Could you check a few things on this drawing? It's one solid part, dimensions in mm from its lowest x, y, z. A direction names the side the tool comes from. Give positions to 0.01 mm unless a question says otherwise; leave off trailing zeros. Order: outer loops, then holes, each group sorted by start corner. A loop starts at its lowest first (then second) coordinate and runs counter-clockwise, first axis right, second up.
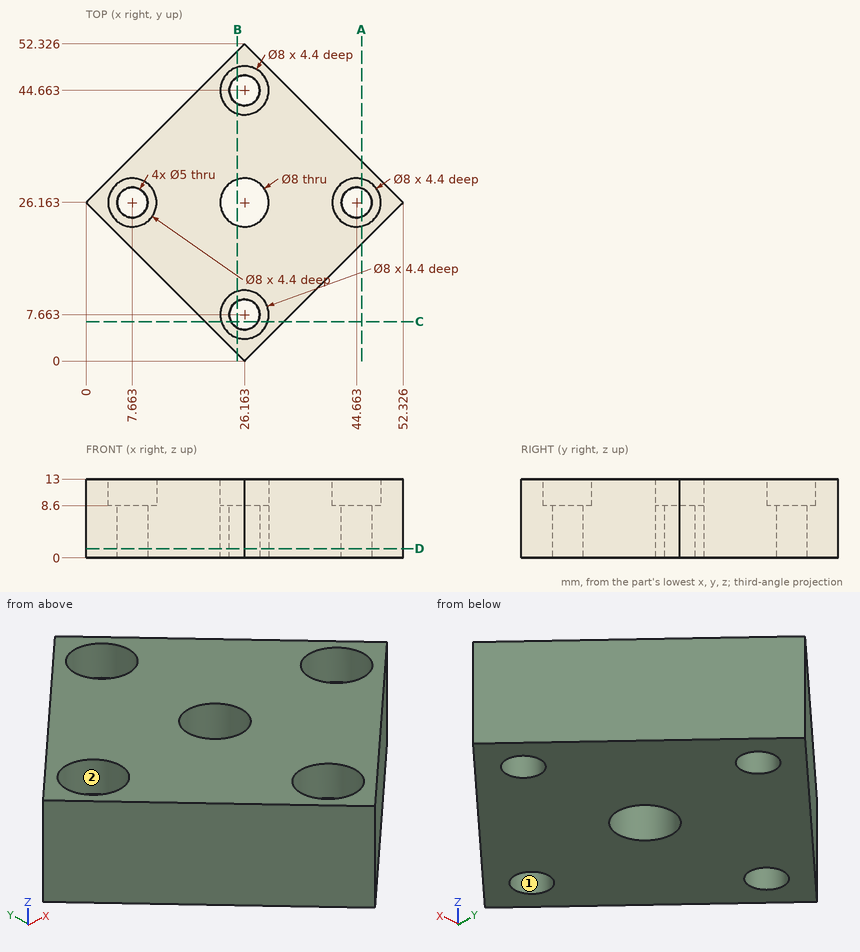
Q1. If we section it at C-C on y = 6.5: List the corners of the cut face in (x, z) for me.
Filled sheet:
outline: (19.66, 0) - (23.95, 0) - (23.95, 8.6) - (22.34, 8.6) - (22.34, 13) - (19.66, 13) - close; (28.38, 0) - (32.66, 0) - (32.66, 13) - (29.99, 13) - (29.99, 8.6) - (28.38, 8.6) - close
Q2. If we section it at B-B on x = 25: List the corners of the cut face in (y, z) for me.
Filled sheet:
outline: (1.16, 0) - (5.45, 0) - (5.45, 8.6) - (3.84, 8.6) - (3.84, 13) - (1.16, 13) - close; (9.88, 0) - (22.34, 0) - (22.34, 13) - (11.49, 13) - (11.49, 8.6) - (9.88, 8.6) - close; (29.99, 0) - (42.45, 0) - (42.45, 8.6) - (40.84, 8.6) - (40.84, 13) - (29.99, 13) - close; (46.88, 0) - (51.16, 0) - (51.16, 13) - (48.49, 13) - (48.49, 8.6) - (46.88, 8.6) - close
Q3. For the marked faces 1 and 2, which set-ups out of +Z, -Z, +X, -X, +Y, -Y let a thin tool reach every point of the face, with its end or its side?
Filled sheet:
face 1: +Z, -Z
face 2: +Z
Q4. If we section it at D-D on z = 1.5: List the corners of the cut face in (x, y) for me, plus the area to 3 significant figures.
Filled sheet:
outline: (0, 26.16) - (26.16, 0) - (52.33, 26.16) - (26.16, 52.33) - close; hole circle Ø5 at (7.66, 26.16); hole circle Ø8 at (26.16, 26.16); hole circle Ø5 at (26.16, 7.66); hole circle Ø5 at (26.16, 44.66); hole circle Ø5 at (44.66, 26.16)
area: 1,240 mm2
Q5. If we section it at A-A on x = 45.5: List the corners of the cut face in (y, z) for me, plus the area to 3 significant figures.
Filled sheet:
outline: (19.34, 0) - (23.81, 0) - (23.81, 8.6) - (22.25, 8.6) - (22.25, 13) - (19.34, 13) - close; (28.52, 0) - (32.99, 0) - (32.99, 13) - (30.07, 13) - (30.07, 8.6) - (28.52, 8.6) - close
area: 103 mm2
Q6. I'm going to push flat-ended pins straight in: P1, Ø4, axis at x = 44, y = 39, coming from the +Z side; P2, Ø2, axis at x = 7, z = 3, coming from the -Y side; P3, Ø2.5, axis at x = 46.5, y = 25, coming from the +Z side; P4, Ø1, axis at x = 46, z = 9.5, coming from the +Y side. Where does each tip first touch, or does it pass through?
Filled sheet:
P1: passes through
P2: stops at y = 18.16
P3: stops at z = 8.6
P4: stops at y = 32.99
Q7. I need wall thicknesses on L1, parallel to Y at x = 29.5, z = 12; L2, parallel to Y at x = 28, z = 2.25; L3, parallel to X at y = 27, z = 2. Which ranges of each line are inside material? Lowest first, please.
Filled sheet:
L1: y = 3.34 to 5.46, 9.87 to 23.96, 28.37 to 42.46, 46.87 to 48.99
L2: y = 1.84 to 5.97, 9.36 to 22.61, 29.72 to 42.97, 46.36 to 50.49
L3: x = 0.84 to 5.31, 10.02 to 22.25, 30.07 to 42.31, 47.02 to 51.49
